from build123d import *

# Parameters (mm, degrees)
MODEL_W             = 15.4
MODEL_H             = 5.4
MODEL_W_2           = 10.4
MODEL_H_2           = 15.4
MODEL_H_3           = 30.4
BOSS_EXTRUDE1_DEPTH = 17


with BuildPart() as part:
    # Model → Boss-Extrude1 (new body)
    with BuildSketch(Plane.XY):
        with BuildLine():
            Line((-144.178149878, -108.319218198), (-99.378149878, -108.319218198))
            Line((-99.378149878, -108.319218198), (-99.378149878, -70.619218198))
            Line((-99.378149878, -70.619218198), (-88.978149878, -70.619218198))
            Line((-88.978149878, -70.619218198), (-88.978149878, -108.319218198))
            Line((-88.978149878, -108.319218198), (50.621850122, -108.319218198))
            Line((50.621850122, -108.319218198), (50.621850122, -70.619218198))
            Line((50.621850122, -70.619218198), (61.021850122, -70.619218198))
            Line((61.021850122, -70.619218198), (61.021850122, -108.319218198))
            Line((61.021850122, -108.319218198), (105.821850122, -108.319218198))
            ThreePointArc((105.821850122, -108.319218198), (119.963985745, -102.461353822), (125.821850122, -88.319218198))
            Line((125.821850122, -88.319218198), (125.821850122, -13.319218198))
            ThreePointArc((125.821850122, -13.319218198), (119.963985745, 0.822917426), (105.821850122, 6.680781802))
            Line((105.821850122, 6.680781802), (85.821850122, 6.680781802))
            ThreePointArc((85.821850122, 6.680781802), (75.215248404, 11.074180084), (70.821850122, 21.680781802))
            Line((70.821850122, 21.680781802), (70.821850122, 101.680781802))
            ThreePointArc((70.821850122, 101.680781802), (75.215248404, 112.28738352), (85.821850122, 116.680781802))
            Line((85.821850122, 116.680781802), (105.821850122, 116.680781802))
            ThreePointArc((105.821850122, 116.680781802), (119.963985745, 122.538646178), (125.821850122, 136.680781802))
            Line((125.821850122, 136.680781802), (125.821850122, 211.680781802))
            ThreePointArc((125.821850122, 211.680781802), (119.963985745, 225.822917426), (105.821850122, 231.680781802))
            Line((105.821850122, 231.680781802), (61.021850122, 231.680781802))
            Line((61.021850122, 231.680781802), (61.021850122, 226.480781802))
            Line((61.021850122, 226.480781802), (48.121850122, 226.480781802))
            Line((48.121850122, 226.480781802), (48.121850122, 231.680781802))
            Line((48.121850122, 231.680781802), (33.521850122, 231.680781802))
            Line((33.521850122, 231.680781802), (33.521850122, 226.480781802))
            Line((33.521850122, 226.480781802), (18.121850122, 226.480781802))
            Line((18.121850122, 226.480781802), (18.121850122, 231.680781802))
            Line((18.121850122, 231.680781802), (3.521850122, 231.680781802))
            Line((3.521850122, 231.680781802), (3.521850122, 226.480781802))
            Line((3.521850122, 226.480781802), (-11.878149878, 226.480781802))
            Line((-11.878149878, 226.480781802), (-11.878149878, 231.680781802))
            Line((-11.878149878, 231.680781802), (-26.478149878, 231.680781802))
            Line((-26.478149878, 231.680781802), (-26.478149878, 226.480781802))
            Line((-26.478149878, 226.480781802), (-41.878149878, 226.480781802))
            Line((-41.878149878, 226.480781802), (-41.878149878, 231.680781802))
            Line((-41.878149878, 231.680781802), (-86.478149878, 231.680781802))
            Line((-86.478149878, 231.680781802), (-86.478149878, 226.480781802))
            Line((-86.478149878, 226.480781802), (-99.378149878, 226.480781802))
            Line((-99.378149878, 226.480781802), (-99.378149878, 231.680781802))
            Line((-99.378149878, 231.680781802), (-144.178149878, 231.680781802))
            ThreePointArc((-144.178149878, 231.680781802), (-158.320285502, 225.822917426), (-164.178149878, 211.680781802))
            Line((-164.178149878, 211.680781802), (-164.178149878, 136.680781802))
            ThreePointArc((-164.178149878, 136.680781802), (-158.320285502, 122.538646178), (-144.178149878, 116.680781802))
            Line((-144.178149878, 116.680781802), (-124.178149878, 116.680781802))
            ThreePointArc((-124.178149878, 116.680781802), (-113.571548161, 112.28738352), (-109.178149878, 101.680781802))
            Line((-109.178149878, 101.680781802), (-109.178149878, 21.680781802))
            ThreePointArc((-109.178149878, 21.680781802), (-113.571548161, 11.074180084), (-124.178149878, 6.680781802))
            Line((-124.178149878, 6.680781802), (-144.178149878, 6.680781802))
            ThreePointArc((-144.178149878, 6.680781802), (-158.320285502, 0.822917426), (-164.178149878, -13.319218198))
            Line((-164.178149878, -13.319218198), (-164.178149878, -88.319218198))
            ThreePointArc((-164.178149878, -88.319218198), (-158.320285502, -102.461353822), (-144.178149878, -108.319218198))
        make_face()
        with Locations((30.321850122, 129.180781802)):
            Rectangle(MODEL_W, MODEL_H, mode=Mode.SUBTRACT)
        with Locations((-68.678149878, 129.180781802)):
            Rectangle(MODEL_W, MODEL_H, mode=Mode.SUBTRACT)
        with Locations((30.321850122, -5.819218198)):
            Rectangle(MODEL_W, MODEL_H, mode=Mode.SUBTRACT)
        with Locations((-68.678149878, -5.819218198)):
            Rectangle(MODEL_W, MODEL_H, mode=Mode.SUBTRACT)
        with Locations((-94.178149878, 206.680781802)):
            Rectangle(MODEL_W_2, MODEL_H_2, mode=Mode.SUBTRACT)
        with Locations((-94.178149878, -25.819218198)):
            Rectangle(MODEL_W_2, MODEL_H_3, mode=Mode.SUBTRACT)
        with Locations((-94.178149878, 94.180781802)):
            Rectangle(MODEL_W_2, MODEL_H_3, mode=Mode.SUBTRACT)
        with Locations((-94.178149878, 154.180781802)):
            Rectangle(MODEL_W_2, MODEL_H_3, mode=Mode.SUBTRACT)
        with Locations((55.821850122, -25.819218198)):
            Rectangle(MODEL_W_2, MODEL_H_3, mode=Mode.SUBTRACT)
        with Locations((55.821850122, 94.180781802)):
            Rectangle(MODEL_W_2, MODEL_H_3, mode=Mode.SUBTRACT)
        with Locations((55.821850122, 154.180781802)):
            Rectangle(MODEL_W_2, MODEL_H_3, mode=Mode.SUBTRACT)
        with Locations((18.321850122, -100.819218198)):
            Rectangle(MODEL_W, MODEL_H, mode=Mode.SUBTRACT)
        with Locations((-56.678149878, -100.819218198)):
            Rectangle(MODEL_W, MODEL_H, mode=Mode.SUBTRACT)
        with Locations((55.821850122, 206.680781802)):
            Rectangle(MODEL_W_2, MODEL_H_2, mode=Mode.SUBTRACT)
        with Locations((-94.178149878, 34.180781802)):
            Rectangle(MODEL_W_2, MODEL_H_3, mode=Mode.SUBTRACT)
    extrude(amount=BOSS_EXTRUDE1_DEPTH)


solid = part.part
Check sheet for the modelled part. Datum: model origin and axes. Units: mm. A direction names the side the tool comes from. Round coordinates to 2 decimals unless told otherwise and drop trailing zeros. Order: outer loops, then holes, each group sorted by start corner. A loop starts at its lowest first (then second) coordinate and runs counter-clockwise, first axis right, second up.
(1) Cross-section at A-A, the plane y = 96.5. Enter the section's corners in (x, z).
(2) Draft check along Y on faces 6 (the flat face through (-94, 214.381, 8)), 7 (the flat face through (-21, 64, 17)), 8 (the flat face through (41, 231.681, 8)), 9 (the flat face through (56, -70.619, 8)). Enter one of: pulls with the +Y half, pulls with the -Y half, needs draft (parallel to the pull), parting line crosses it, or undercut.
(3) Scan lines: probe 1 along X at (y, z) = (-85, 7.25); probe 2 along X at (y, z) = (102, 11.75); probe 3 along Y at (x, z) = (-66.5, 14). Record each from-to range of solid material in increasing order.
(4) Cross-section at C-C, the plane y = -75. Enter the section's corners in (x, z).
(5) Cross-section at B-B, the plane z = 10. State how many separate pieces and enclosed holes the cut face has, and give its area (3 significant figures).
(6) Go/stop test with flat-tipped pins: P1, Ø3, axis at x = -96.5, z = 4.5, coming from the -Y side; P2, Ø5, axis at y = 96.5, z = 12.5, coming from the +X side; P3, Ø4, axis at y = 229, z = 9, coming from the +X side. Record where each tip stops, or that it passes through.
(7) Access from +Z, -Z, +X, -X, +Y, -Y to the whole of each face (thin tool, end or side, straight path). Record for faces 1 (the flat face through (56, 214.381, 8)), 2 (the flat face through (-88.978, -89, 8)), 3 (the cylindrical face through (-113.456, 11.191, 8.381)), 4 (the cylindrical face through (120.119, 0.667, 8.381)), 5 (the flat face through (55, 226.481, 8)).
Check sheet entries:
1. outline: (-109.18, 0) - (-99.38, 0) - (-99.38, 17) - (-109.18, 17) - close; (-88.98, 0) - (50.62, 0) - (50.62, 17) - (-88.98, 17) - close; (61.02, 0) - (70.82, 0) - (70.82, 17) - (61.02, 17) - close
2. face 6: undercut
2. face 7: needs draft
2. face 8: pulls with the +Y half
2. face 9: pulls with the -Y half
3. probe 1: x = -164.18 to -99.38, -88.98 to 50.62, 61.02 to 125.82
3. probe 2: x = -109.18 to -99.38, -88.98 to 50.62, 61.02 to 70.83
3. probe 3: y = -108.32 to -8.52, -3.12 to 126.48, 131.88 to 231.68
4. outline: (-164.18, 0) - (-99.38, 0) - (-99.38, 17) - (-164.18, 17) - close; (-88.98, 0) - (50.62, 0) - (50.62, 17) - (-88.98, 17) - close; (61.02, 0) - (125.82, 0) - (125.82, 17) - (61.02, 17) - close
5. separate pieces: 1
5. enclosed holes: 15
5. area: 81,800 mm2
6. P1: stops at y = -70.62
6. P2: stops at x = 70.82
6. P3: stops at x = 118.68
7. face 1: +Z, -Z
7. face 2: +Z, -Z, -Y
7. face 3: +Z, -Z, -X
7. face 4: +Z, -Z, +X
7. face 5: +Z, -Z, +Y
